```python
from build123d import *

# Parameters (mm, degrees)
F0_W     = 500
F0_H     = 250
F1_DEPTH = 250
F3_DEPTH = 110.811708
F6_D     = 100


with BuildPart() as f1:
    # F0 (on Top) → F1 (new body)
    with BuildSketch(Plane.XY):
        Rectangle(F0_W, F0_H)
    extrude(amount=-F1_DEPTH)

    # F2 (on face) → F3 (join)
    with BuildSketch(Plane.YZ.offset(250)):
        with BuildLine():
            Line((50, -125), (125, -125))
            Line((125, -125), (125, 0))
            Line((125, 0), (0, 0))
            Line((0, 0), (0, -75))
            ThreePointArc((0, -75), (35.355339, -89.644661), (50, -125))
        make_face()
        with BuildLine():
            Line((0, -125), (50, -125))
            ThreePointArc((50, -125), (35.355339, -89.644661), (0, -75))
            Line((0, -75), (0, -125))
        make_face()
        with BuildLine():
            ThreePointArc((0, -175), (35.355339, -160.355339), (50, -125))
            Line((50, -125), (0, -125))
            Line((0, -125), (0, -175))
        make_face()
        with BuildLine():
            Line((125, -250), (125, -125))
            Line((125, -125), (50, -125))
            ThreePointArc((50, -125), (35.355339, -160.355339), (0, -175))
            Line((0, -175), (0, -250))
            Line((0, -250), (125, -250))
        make_face()
    extrude(amount=-F3_DEPTH)

    # F6 (through all)
    with Locations(Plane.YZ.offset(250)):
        with Locations((0, -125)):
            Hole(F6_D / 2)


solid = f1.part
```
Model file for the job. Use its own axes, mm. Give positions to 0.01 mm unless a question says otherwise; leave off trailing zeros. Write each loop counter-clockwise with the first axis right and the second up, starting at its lowest first coordinate (ties: lowest second). Pieces come first, ordered by that corner, then holes. Notation, with made-up numbers: (-34, 36) - (-5, 36) arc R19 cw to (-5, 45) - close; hole circle Ø9 at (55.5, -14.5). An arc over 180 degrees is marked (long way). One line per question, with ' | ' between items. Start each with the question number.
(1) Two-plate mould, pull along Y, no slides. Class faces 1 (the face through (-3, -125, -123)), 2 (the face through (-3.5, -47.69, -109.98)), 3 (the face through (-250, -2, -68)): +Y half, -Y half, draft (parallel to the pull), parting line (faces both ways), or undercut.
(2) Slice it at C-C on x = -63.5. Write the cut outline in (y, z).
(3) Slice it at B-B on y = 0. Write the cut outline in (x, z).
(4) Slice it at A-A on z = -125. Write the cut outline in (x, y), plus the area to 3 significant figures.
(5) Wall check: line 1 along Z through (x, y) = (-173, 1.5); line 2 along Z through (x, y) = (28, -22.5); line 3 along Y through (x, z) = (-172.5, -132). Give the ranges that are in metal, low to high. Write a range as from..to.
Results below:
1) face 1: -Y half | face 2: undercut | face 3: draft
2) outline: (-125, -250) - (125, -250) - (125, 0) - (-125, 0) - close; hole circle Ø100 at (0, -125)
3) outline: (-250, -250) - (250, -250) - (250, -175) - (-250, -175) - close; (-250, -75) - (250, -75) - (250, 0) - (-250, 0) - close
4) outline: (-250, -125) - (250, -125) - (250, -50) - (-250, -50) - close; (-250, 50) - (250, 50) - (250, 125) - (-250, 125) - close | area: 75,000 mm^2
5) line 1: -250..-174.98, -75.02..0 | line 2: -250..-169.65, -80.35..0 | line 3: -125..-49.51, 49.51..125
